Geometry check sheet. Reference: the model listing, model coordinates, mm. Face numbers are marked on the shaded views. A direction names the side the tool comes from. Give positions to 0.01 mm unless a question says otherwise; leave off trailing zeros. Order: outer loops, then holes, each group sorted by start corner. A loop starts at its lowest first (then second) coordinate and runs counter-clockwise, first axis right, second up. Notation, with made-up numbers: M 88.5,2.5 L 141.5,2.5 A21 cw 141.5,10.5 Z; hole C 59,47 d1. An arc over 180 degrees is marked long. Put each result on its own line as item: value. Start each with the question number.
Q1. Mould release check, pull along Z, two halves, no side actions. Record for the marked faces 1, 2 and 3: +Z half, -Z half, draft (parallel to the pull), parting line (faces both ways), or undercut.
Q2. Section check C-C on y = -1.5. Record the cut outline in (x, z), then the cut area to 3 significant figures.
Q3. Section check A-A on y = 7. Record the cut outline in (x, z) (3 decimals), then the cut area to 3 significant figures.
Q4. Material ranges on L1, parallel to X at y = 6.75, z = -11.5; L2, parallel to Z at x = -8, y = 8.75; L3, parallel to Y at x = -10.5, z = 20.5, recorded low to high.
Q5. Section check B-B on z = 0. Record the cut outline in (x, y).
Q6. Go/stop test with flat-tipped pins: pin 1 (3.5 mm diameter, centred on x = 2, y = 13.5, fed in from +Z); pin 2 (1.5 mm diameter, centred on y = 7, z = -19.5, fed in from -X); pin 3 (2 mm diameter, centred on x = 0.5, z = -19.5, fed in from -Y). Record where each tip stops, or that it passes through.
Q7. Access from +Z, -Z, +X, -X, +Y, -Y to the whole of each face (thin tool, end or side, straight path). Record for the marked faces 4 and 5.
Q8. Section check D-D on x = 16. Record the cut outline in (y, z), then the cut area to 3 significant figures.
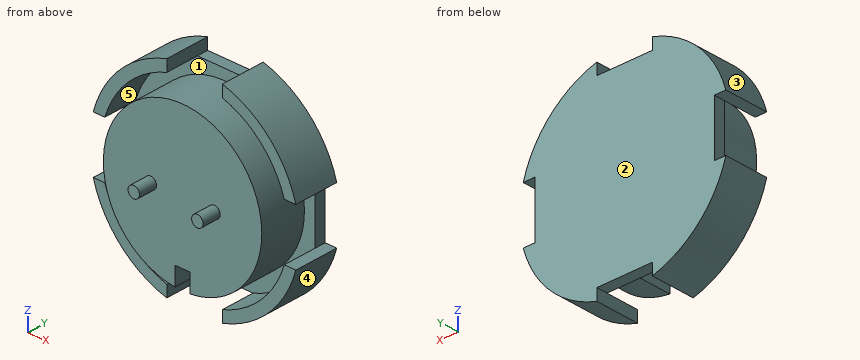
```python
from build123d import *

# Parameters (mm, degrees)
SKETCH1_R                = 1.55
BOSS_EXTRUDE1_DEPTH      = 11.5
SKETCH1_3_R              = 1.55
BOSS_EXTRUDE2_DEPTH      = 11.5
BOSS_EXTRUDE2_DEPTH_BACK = 5
BOSS_EXTRUDE3_START      = 11.5
SKETCH2_R                = 21.4
SKETCH2_R_2              = 18.4
BOSS_EXTRUDE3_DEPTH      = 4
BOSS_EXTRUDE4_START      = 15.5
SKETCH2_3_R              = 21.4
BOSS_EXTRUDE4_DEPTH      = 3
BOSS_EXTRUDE5_START      = 15.5
BOSS_EXTRUDE5_DEPTH      = 12


with BuildPart() as part:
    # Sketch1 → Boss-Extrude1 (new body)
    with BuildSketch(Plane(origin=(0, 0, 0), x_dir=(1, 0, 0), z_dir=(0, 1, 0))):
        with BuildLine():
            Line((2.05, 16.301584448), (-2.05, 16.301584448))
            Line((-2.05, 16.301584448), (-2.05, 21.301584448))
            ThreePointArc((-2.05, 21.301584448), (0, -21.4), (2.05, 21.301584448))
            Line((2.05, 21.301584448), (2.05, 16.301584448))
        make_face()
        with Locations(Location((-8.6, 0, 0), (0, 0, 270))):
            Circle(SKETCH1_R, mode=Mode.SUBTRACT)
        with Locations(Location((8.6, 0, 0), (0, 0, 270))):
            Circle(SKETCH1_R, mode=Mode.SUBTRACT)
    extrude(amount=BOSS_EXTRUDE1_DEPTH)

    # Sketch1<3> → Boss-Extrude2 (add, two sides)
    with BuildSketch(Plane(origin=(0, 0, 0), x_dir=(1, 0, 0), z_dir=(0, 1, 0))) as boss_extrude2_sk:
        with Locations(Location((-8.6, 0, 0), (0, 0, 270))):
            Circle(SKETCH1_3_R)
        with Locations(Location((8.6, 0, 0), (0, 0, 270))):
            Circle(SKETCH1_3_R)
    extrude(amount=BOSS_EXTRUDE2_DEPTH)
    extrude(boss_extrude2_sk.sketch, amount=-BOSS_EXTRUDE2_DEPTH_BACK)

    # Sketch2 → Boss-Extrude3 (add)
    with BuildSketch(Plane(origin=(0, 0, 0), x_dir=(1, 0, 0), z_dir=(0, 1, 0)).offset(BOSS_EXTRUDE3_START)):
        with Locations(Location((0, 0, 0), (0, 0, 84.502956314))):
            Circle(SKETCH2_R)
        Circle(SKETCH2_R_2, mode=Mode.SUBTRACT)
        Circle(SKETCH2_R_2)
    extrude(amount=BOSS_EXTRUDE3_DEPTH)

    # Sketch2<3> → Boss-Extrude4 (add)
    with BuildSketch(Plane(origin=(0, 0, 0), x_dir=(1, 0, 0), z_dir=(0, 1, 0)).offset(BOSS_EXTRUDE4_START)):
        with BuildLine():
            Line((7.5, 24.241299986), (-7.5, 24.241299986))
            ThreePointArc((-7.5, 24.241299986), (-17.942834573, 17.942834573), (-24.241299986, 7.5))
            Line((-24.241299986, 7.5), (-24.241299986, -7.5))
            ThreePointArc((-24.241299986, -7.5), (-17.942834573, -17.942834573), (-7.5, -24.241299986))
            Line((-7.5, -24.241299986), (7.5, -24.241299986))
            ThreePointArc((7.5, -24.241299986), (17.942834573, -17.942834573), (24.241299986, -7.5))
            Line((24.241299986, -7.5), (24.241299986, 7.5))
            ThreePointArc((24.241299986, 7.5), (17.942834573, 17.942834573), (7.5, 24.241299986))
        make_face()
        with Locations(Location((0, 0, 0), (0, 0, 84.502956314))):
            Circle(SKETCH2_3_R, mode=Mode.SUBTRACT)
    extrude(amount=-BOSS_EXTRUDE4_DEPTH)

    # Sketch2<4> → Boss-Extrude5 (add)
    with BuildSketch(Plane(origin=(0, 0, 0), x_dir=(1, 0, 0), z_dir=(0, 1, 0)).offset(BOSS_EXTRUDE5_START)):
        with BuildLine():
            Line((-7.5, 24.241299986), (-7.5, 27.365866056))
            ThreePointArc((-7.5, 27.365866056), (-20.064154916, 20.064154916), (-27.365866056, 7.5))
            Line((-27.365866056, 7.5), (-24.241299986, 7.5))
            ThreePointArc((-24.241299986, 7.5), (-17.942834573, 17.942834573), (-7.5, 24.241299986))
        make_face()
        with BuildLine():
            ThreePointArc((27.365866056, 7.5), (20.064154916, 20.064154916), (7.5, 27.365866056))
            Line((7.5, 27.365866056), (7.5, 24.241299986))
            ThreePointArc((7.5, 24.241299986), (17.942834573, 17.942834573), (24.241299986, 7.5))
            Line((24.241299986, 7.5), (27.365866056, 7.5))
        make_face()
        with BuildLine():
            Line((-24.241299986, -7.5), (-27.365866056, -7.5))
            ThreePointArc((-27.365866056, -7.5), (-20.064154916, -20.064154916), (-7.5, -27.365866056))
            Line((-7.5, -27.365866056), (-7.5, -24.241299986))
            ThreePointArc((-7.5, -24.241299986), (-17.942834573, -17.942834573), (-24.241299986, -7.5))
        make_face()
        with BuildLine():
            Line((27.365866056, -7.5), (24.241299986, -7.5))
            ThreePointArc((24.241299986, -7.5), (17.942834573, -17.942834573), (7.5, -24.241299986))
            Line((7.5, -24.241299986), (7.5, -27.365866056))
            ThreePointArc((7.5, -27.365866056), (20.064154916, -20.064154916), (27.365866056, -7.5))
        make_face()
    extrude(amount=-BOSS_EXTRUDE5_DEPTH)


solid = part.part
```
Results found:
1. face 1: undercut
1. face 2: draft
1. face 3: +Z half
2. outline: C -8.6,0 d3.1; C 8.6,0 d3.1
2. area: 15.1 mm^2
3. outline: M -27.366,-7.5 A28.375 ccw -7.5,-27.366 L -7.5,-24.241 A25.375 cw -24.241,-7.5 Z; M -27.366,7.5 L -24.241,7.5 A25.375 cw -7.5,24.241 L -7.5,27.366 A28.375 ccw Z; M -2.05,-21.302 L -2.05,-16.302 L 2.05,-16.302 L 2.05,-21.302 A21.4 ccw long Z; M 7.5,-27.366 A28.375 ccw 27.366,-7.5 L 24.241,-7.5 A25.375 cw 7.5,-24.241 Z; M 7.5,24.241 A25.375 cw 24.241,7.5 L 27.366,7.5 A28.375 ccw 7.5,27.366 Z
3. area: 1,740 mm^2
4. L1: x = -25.94 to -22.62, -18.05 to 18.05, 22.62 to 25.94
4. L2: z = -27.22 to -24.08, -19.85 to 19.85, 24.08 to 27.22
4. L3: y = 12.5 to 15.5
5. outline: M -24.24,12.5 L -21.4,12.5 L -21.4,0 L -10.15,0 L -10.15,-5 L -7.05,-5 L -7.05,0 L 7.05,0 L 7.05,-5 L 10.15,-5 L 10.15,0 L 21.4,0 L 21.4,12.5 L 24.24,12.5 L 24.24,15.5 L -24.24,15.5 Z
6. pin 1: stops at z = 24.24
6. pin 2: stops at x = -21.3
6. pin 3: stops at y = 11.5
7. face 4: -Z, +X, +Y, -Y
7. face 5: -Y
8. outline: M 0,-14.21 L 12.5,-14.21 L 12.5,-19.69 L 3.5,-19.69 L 3.5,-23.43 L 15.5,-23.43 L 15.5,23.43 L 3.5,23.43 L 3.5,19.69 L 12.5,19.69 L 12.5,14.21 L 0,14.21 Z
8. area: 563 mm^2
